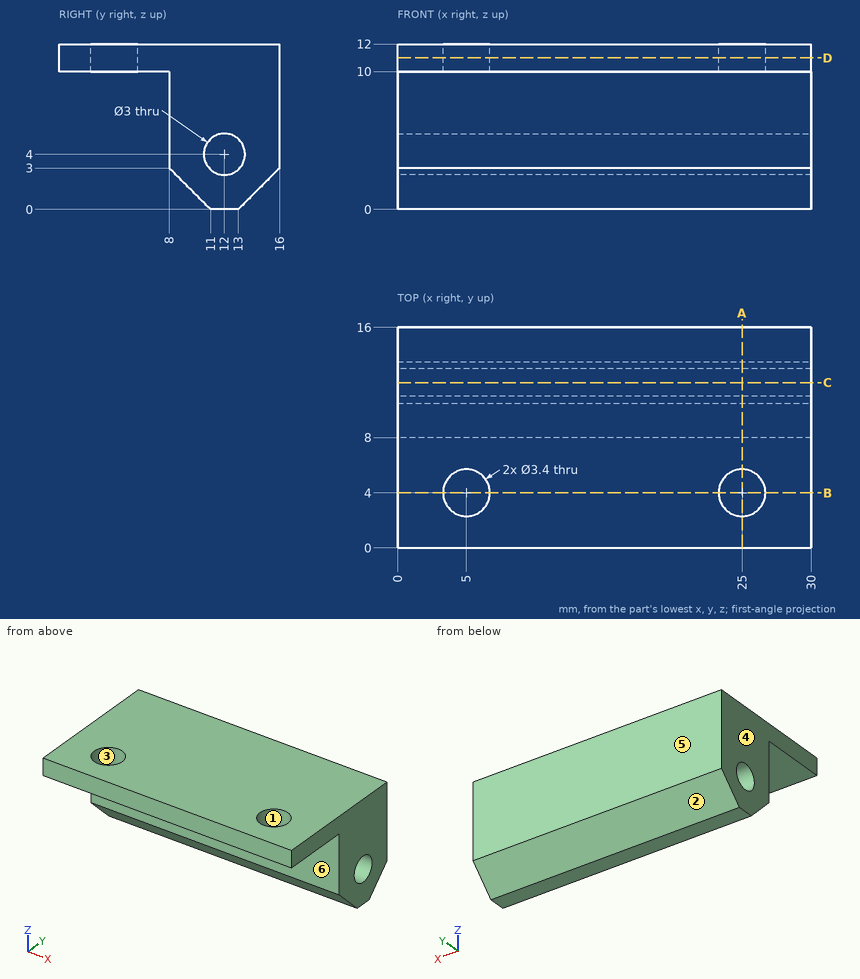
Design review of the part shown in the three views and the two pictorial views. Dimensions are in mm from the part's minimum x, y and z. A direction names the side the tool comes from. Give positions to 0.01 mm unless a question says otherwise; leave off trailing zeros. Loops run counter-clockwise (first coordinate to the right, second up) from the corner with the lowest first, then second, coordinate; pieces in that order, holes last. Notation, with made-up numbers: (-26, 61.25) - (-21, 61.25) arc R14 ccw to (-21, 66.25) - close; hole circle Ø3 at (50, 55.5). An arc over 180 degrees is marked (long way). Use CSV: the item, a comma, the result in double quotes. Start each with the question number.
1. Insertion check: P1, Ø2.5, axis at x = 5, y = 4, coming from the -Z side; P2, Ø9, axis at x = 7.5, y = 3, coming from the -Z side; P3, Ø1.5, axis at x = 9, z = 2, coming from the -Y side; P4, Ø6, axis at y = 5.5, z = 7, coming from the -X side. Each pin has a flat end and moves straight along its axis. Give the tip position at first contact, or say it passes through.
2. Draft analysis for pull direction Y (two halves, no side actions). For the marked faces 1, 2, 3 and 4, state which applies: released by +Y, released by -Y, zero draft, split by the parting line, or undercut.
3. Add section B-B (y = 4). State the section outline as (x, z) points.
4. Add section C-C (y = 12). State the section outline as (x, z) points, plus the area to 3 significant figures.
5. Wall thickness on L1, parallel to Y at x = 25, z = 4; L2, parallel to Y at x = 25, z = 11.1; L3, parallel to Y at x = 12, z = 8.25: over which ranges is each line inside the solid? List them lowest first.
6. Add section A-A (x = 25). State the section outline as (y, z) points.
7. Add section D-D (z = 11). State the section outline as (x, y) points, plus the area to 3 significant figures.
8. Machinability: for the marked faces 5 and 6, which of the approach directions +Z, -Z, +X, -X, +Y, -Y give a long, thin tool a straight path to every point of the face, cutting with its end or side? Answer none if there is none.
Results found:
1,P1,"passes through"
1,P2,"stops at z = 10"
1,P3,"stops at y = 8.25"
1,P4,"stops at x = 0"
2,face 1,"undercut"
2,face 2,"released by +Y"
2,face 3,"undercut"
2,face 4,"zero draft"
3,outline,"(0, 10) - (3.3, 10) - (3.3, 12) - (0, 12) - close; (6.7, 10) - (23.3, 10) - (23.3, 12) - (6.7, 12) - close; (26.7, 10) - (30, 10) - (30, 12) - (26.7, 12) - close"
4,outline,"(0, 0) - (30, 0) - (30, 2.5) - (0, 2.5) - close; (0, 5.5) - (30, 5.5) - (30, 12) - (0, 12) - close"
4,area,"270 mm²"
5,L1,"y = 8 to 10.5, 13.5 to 16"
5,L2,"y = 0 to 2.3, 5.7 to 16"
5,L3,"y = 8 to 16"
6,outline,"(0, 10) - (2.3, 10) - (2.3, 12) - (0, 12) - close; (5.7, 10) - (8, 10) - (8, 3) - (11, 0) - (13, 0) - (16, 3) - (16, 12) - (5.7, 12) - close; hole circle Ø3 at (12, 4)"
7,outline,"(0, 0) - (30, 0) - (30, 16) - (0, 16) - close; hole circle Ø3.4 at (5, 4); hole circle Ø3.4 at (25, 4)"
7,area,"462 mm²"
8,face 5,"+Z, -Z, +X, -X, +Y"
8,face 6,"-Z, +X, -X, -Y"
